Part print with two shaded views. Sizes in mm from the minimum x, y, z corner. Coordinates: 2 decimals unless noted, no trailing zeros. Loops run counter-clockwise (first coordinate to the right, second up) from the corner with the lowest first, then second, coordinate; pieces in that order, holes last.
Item 1: Cut at A-A (y = 115.75). List the corners of the cut face in (x, z).
Item 2: Cut at C-C (z = 9). Count the separate pieces of the cut face and the enclosed holes in it, and give its area (3 significant figures).
Item 3: Cut at B-B (x = 142.5). List the corners of the cut face in (y, z).
Item 4: Mould opens along Z. For the marked faces 1, 2 and 3 say: released by +Z, released by -Z, zero draft, split by the parting line, or undercut.
Item 5: Drill centre lines: line 1 along Y through (x, z) = (115.75, 5.5); line 2 along Y through (x, z) = (186, 5.5) (1 decimal); line 3 along X through (y, z) = (124, 5) (1 decimal). Where is each one in solid material? Low to high.
Item 6: Flat gauge pins, fed straight in: pin 1 (1.5 mm diameter, centred on x = 147, z = 10, fed in from -Y); pin 2 (5 mm diameter, centred on x = 82, z = 12, fed in from -Y); pin 3 (4 mm diameter, centred on y = 166, z = 5, fed in from +X) (1 decimal). Where does each tip first touch, or does it go through?
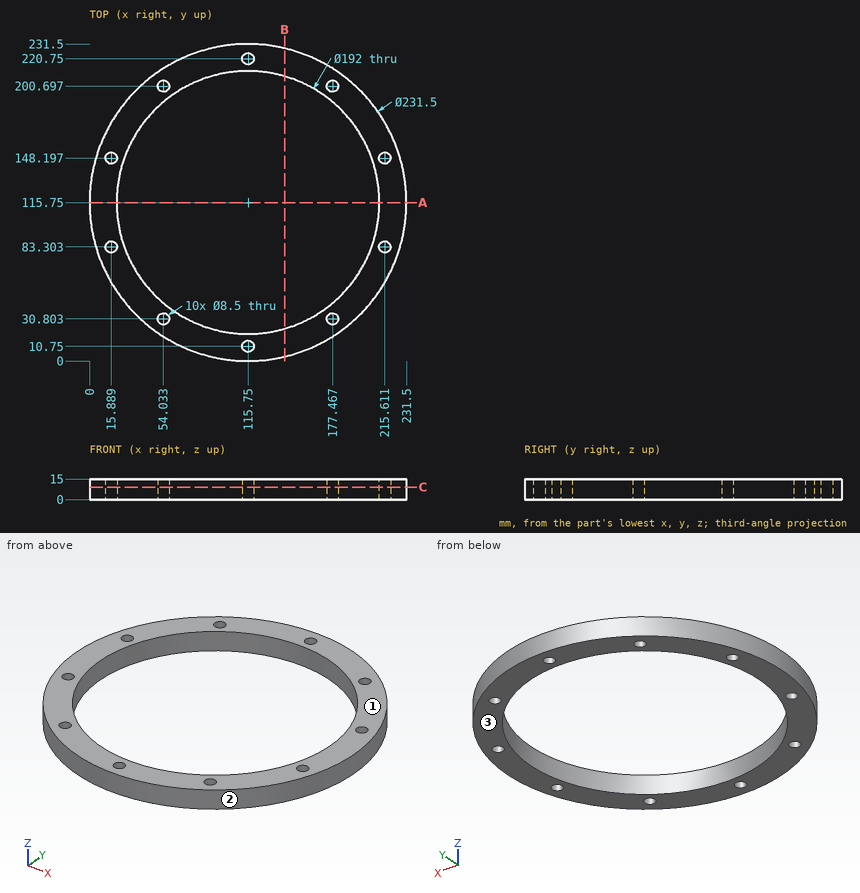
Filled sheet:
1. outline: (0, 0) - (19.75, 0) - (19.75, 15) - (0, 15) - close; (211.75, 0) - (231.5, 0) - (231.5, 15) - (211.75, 15) - close
2. separate pieces: 1
2. enclosed holes: 11
2. area: 12,600 mm2
3. outline: (3.13, 0) - (23.55, 0) - (23.55, 15) - (3.13, 15) - close; (207.95, 0) - (228.37, 0) - (228.37, 15) - (207.95, 15) - close
4. face 1: released by +Z
4. face 2: zero draft
4. face 3: released by -Z
5. line 1: y = 0 to 6.5, 15 to 19.75, 211.75 to 216.5, 225 to 231.5
5. line 2: y = 23.8 to 50.3, 181.2 to 207.7
5. line 3: x = 0.3 to 20.1, 211.4 to 231.2
6. pin 1: stops at y = 4.09
6. pin 2: stops at y = 4.3
6. pin 3: stops at x = 221
